Source: CAD feature listing. Evaluate the final solid. Frame: model axes, mm. Give positions to 0.01 mm unless a question says otherwise; leave off trailing zeros. Order: outer loops, then holes, each group sorted by start corner. A loop starts at its lowest first (then second) coordinate and runs counter-clockwise, first axis right, second up. Notation, with made-up numbers: (19, 29.5) -> (57, 29.5) arc R29 ccw to (57, 61.5) -> close; hole circle Ø6 at (-12, 13.25). An arc over 180 degrees is marked (long way). Answer in a Markdown table with one row per item.
```python
from build123d import *

# Parameters (mm, degrees)
SKETCH1_R           = 20
SKETCH1_R_2         = 2.75
BOSS_EXTRUDE1_DEPTH = 2.5
CUT_EXTRUDE3_DEPTH  = 2.5
SKETCH4_R           = 1.25
CUT_EXTRUDE4_DEPTH  = 5
SKETCH2_R           = 3
SKETCH2_R_2         = 2.75
BOSS_EXTRUDE2_DEPTH = 5


with BuildPart() as part:
    # Sketch1 → Boss-Extrude1 (new body)
    with BuildSketch(Plane(origin=(0, 0, 0), x_dir=(1, 0, 0), z_dir=(0, 1, 0))):
        Circle(SKETCH1_R)
        Circle(SKETCH1_R_2, mode=Mode.SUBTRACT)
    extrude(amount=BOSS_EXTRUDE1_DEPTH)

    # Sketch3 → Cut-Extrude3 (cut)
    with BuildSketch(Plane.XZ):
        Polygon((-5.161329605, 1.721273866), (-8.071331697, 3.318997608), (-10.910002092, 1.597723742), (-10.838670395, -1.721273866), (-7.928668303, -3.318997608), (-5.089997908, -1.597723742), align=None)
        Polygon((5.161329605, -1.721273866), (8.071331697, -3.318997608), (10.910002092, -1.597723742), (10.838670395, 1.721273866), (7.928668303, 3.318997608), (5.089997908, 1.597723742), align=None)
    extrude(amount=-CUT_EXTRUDE3_DEPTH, mode=Mode.SUBTRACT)

    # Sketch4 → Cut-Extrude4 (cut)
    with BuildSketch(Plane(origin=(0, 2.5, 0), x_dir=(1, 0, 0), z_dir=(0, 1, 0))):
        with Locations((0, 17)):
            Circle(SKETCH4_R)
        with Locations((0, 20)):
            Circle(SKETCH4_R)
    extrude(amount=-CUT_EXTRUDE4_DEPTH, mode=Mode.SUBTRACT)

    # Sketch2 → Boss-Extrude2 (add)
    with BuildSketch(Plane(origin=(0, 2.5, 0), x_dir=(1, 0, 0), z_dir=(0, 1, 0))):
        Circle(SKETCH2_R)
        Circle(SKETCH2_R_2, mode=Mode.SUBTRACT)
    extrude(amount=BOSS_EXTRUDE2_DEPTH)

    # Mirror7: part across plane


with BuildPart() as part_1:
    add(part.part)
    add(part.part.mirror(Plane.ZX.offset(7.5)))


solid = part_1.part
```
(1) Section query D-D (x = -13). Return the cut outline in (y, z).
A:
| item | result |
|---|---|
| outline | (0, -15.2) -> (2.5, -15.2) -> (2.5, 15.2) -> (0, 15.2) -> close; (12.5, -15.2) -> (15, -15.2) -> (15, 15.2) -> (12.5, 15.2) -> close |
(2) Pull-direction query (Z, two-part tool) for faces 1 (the flat face through (4, 0, 0)), 2 (the flat face through (6.6, 1.23, -2.51)), 3 (the cylindrical face through (-0.03, 1.27, -18.75)); classes: +Z half, -Z half, draft (parallel to the pull), parting line (faces both ways), or undercut.
A:
| item | result |
|---|---|
| face 1 | draft |
| face 2 | undercut |
| face 3 | -Z half |
(3) Section query B-B (y = 2). Return the cut outline in (x, z).
A:
| item | result |
|---|---|
| outline | (-1.25, -19.96) arc R1.25 cw to (1.25, -19.96) arc R20 ccw (long way) to start; hole (-10.91, 1.6) -> (-10.84, -1.72) -> (-7.93, -3.32) -> (-5.09, -1.6) -> (-5.16, 1.72) -> (-8.07, 3.32) -> close; hole circle Ø5.5 at (0, 0); hole circle Ø2.5 at (0, -17); hole (5.09, 1.6) -> (5.16, -1.72) -> (8.07, -3.32) -> (10.91, -1.6) -> (10.84, 1.72) -> (7.93, 3.32) -> close |
(4) First-contact query: pin 1 Ø2 at (x, z) = (0, -17) entering from -Y; pin 2 Ø3 at (y, z) = (2, -5) entering from -X. Flat tips, straight axial feed; report the tip coordinate or a pass-through.
A:
| item | result |
|---|---|
| pin 1 | passes through |
| pin 2 | stops at x = -19.69 |
(5) Ray query, probe 1 along Z at (x, y) = (0, 1.1); probe 2 along Y at (x, z) = (14, 3); probe 3 along X at (y, z) = (10, 0). Return the intervals inside material, ascending.
A:
| item | result |
|---|---|
| probe 1 | z = -18.75 to -18.25, -15.75 to -2.75, 2.75 to 20 |
| probe 2 | y = 0 to 2.5, 12.5 to 15 |
| probe 3 | x = -3 to -2.75, 2.75 to 3 |
(6) Section query A-A (x = 0). Return the cut outline in (y, z).
A:
| item | result |
|---|---|
| outline | (0, -18.75) -> (2.5, -18.75) -> (2.5, -18.25) -> (0, -18.25) -> close; (0, -15.75) -> (2.5, -15.75) -> (2.5, -3) -> (12.5, -3) -> (12.5, -15.75) -> (15, -15.75) -> (15, -2.75) -> (0, -2.75) -> close; (0, 2.75) -> (15, 2.75) -> (15, 20) -> (12.5, 20) -> (12.5, 3) -> (2.5, 3) -> (2.5, 20) -> (0, 20) -> close; (12.5, -18.75) -> (15, -18.75) -> (15, -18.25) -> (12.5, -18.25) -> close |
(7) Section query C-C (z = -13). Return the cut outline in (x, y), plus the area to 3 significant figures.
A:
| item | result |
|---|---|
| outline | (-15.2, 0) -> (15.2, 0) -> (15.2, 2.5) -> (-15.2, 2.5) -> close; (-15.2, 12.5) -> (15.2, 12.5) -> (15.2, 15) -> (-15.2, 15) -> close |
| area | 152 mm^2 |
